Build history of the part. All positions in model axes, mm. A direction names the side the tool comes from. Round coordinates to 2 decimals unless told otherwise and drop trailing zeros. Loops run counter-clockwise (first coordinate to the right, second up) from the corner with the lowest first, then second, coordinate; pieces in that order, holes last. Notation, with made-up numbers: (89.5, 19.25) - (129.5, 19.25) arc R37 ccw to (129.5, 55.25) - close; hole circle Ø4 at (-18, 17.25). An arc over 180 degrees is marked (long way). Use a Markdown table: item, result.
from build123d import *
from build123d.topology import SkipClean

# Parameters (mm, degrees)
BOSS_EXTRUDE1_DEPTH = 2
SKETCH4_R           = 1
CUT_EXTRUDE3_DEPTH  = 2
SKETCH5_R           = 2
CUT_EXTRUDE4_DEPTH  = 1
SKETCH2_R           = 5
CUT_EXTRUDE1_DEPTH  = 10
SKETCH3_R           = 24
CUT_EXTRUDE2_DEPTH  = 10
BOSS_EXTRUDE2_START = 7.2
SKETCH6_R           = 28
SKETCH6_R_2         = 24
BOSS_EXTRUDE2_DEPTH = 7.2
SKETCH7_R           = 28
SKETCH7_R_2         = 14
BOSS_EXTRUDE3_DEPTH = 2
SKETCH9_W           = 14
SKETCH9_H           = 12
BOSS_EXTRUDE4_DEPTH = 4
FILLET1_R           = 7
SKETCH10_R          = 3.25
CUT_EXTRUDE6_DEPTH  = 3
BOSS_EXTRUDE5_DEPTH = 2
FILLET2_R           = 7
FILLET3_R           = 7
FILLET4_R           = 4
FILLET5_R           = 4
SKETCH12_W          = 15
SKETCH12_H          = 7
CUT_EXTRUDE7_DEPTH  = 10


# Some blends are built 0.0001 mm under size
with BuildPart() as part:
    # Sketch1 → Boss-Extrude1 (new body)
    with BuildSketch(Plane(origin=(0, 0, 0), x_dir=(1, 0, 0), z_dir=(0, 1, 0))):
        with BuildLine():
            Line((-37.46998799, 30), (37.46998799, 30))
            ThreePointArc((37.46998799, 30), (0, -48), (-37.46998799, 30))
        make_face()
    extrude(amount=BOSS_EXTRUDE1_DEPTH)

    # Sketch4 → Cut-Extrude3 (cut)
    with BuildSketch(Plane(origin=(0, 2, 0), x_dir=(1, 0, 0), z_dir=(0, 1, 0))):
        with Locations(Location((-44.167045026, 13, 0), (0, 0, 270))):
            Circle(SKETCH4_R)
        with Locations(Location((0, -46.347801012, 0), (0, 0, 270))):
            Circle(SKETCH4_R)
        with Locations(Location((44.167045026, 13, 0), (0, 0, 270))):
            Circle(SKETCH4_R)
    extrude(amount=-CUT_EXTRUDE3_DEPTH, mode=Mode.SUBTRACT)

    # Sketch5 → Cut-Extrude4 (cut)
    with BuildSketch(Plane(origin=(0, 2, 0), x_dir=(1, 0, 0), z_dir=(0, 1, 0))):
        with Locations((-44.167045026, 13)):
            Circle(SKETCH5_R)
        with Locations((0, -46.347801012)):
            Circle(SKETCH5_R)
        with Locations((44.167045026, 13)):
            Circle(SKETCH5_R)
    extrude(amount=-CUT_EXTRUDE4_DEPTH, mode=Mode.SUBTRACT)

    # Sketch2 → Cut-Extrude1 (cut)
    with BuildSketch(Plane(origin=(0, 2, 0), x_dir=(1, 0, 0), z_dir=(0, 1, 0))):
        with Locations(Location((1.35, 0.05, 0), (0, 0, 270))):
            Circle(SKETCH2_R)
    extrude(amount=-CUT_EXTRUDE1_DEPTH, mode=Mode.SUBTRACT)

    # Sketch3 → Cut-Extrude2 (cut)
    with BuildSketch(Plane(origin=(0, 2, 0), x_dir=(1, 0, 0), z_dir=(0, 1, 0))):
        with Locations(Location((1.35, 0.05, 0), (0, 0, 270))):
            Circle(SKETCH3_R)
    extrude(amount=-CUT_EXTRUDE2_DEPTH, mode=Mode.SUBTRACT)

    # Sketch6 → Boss-Extrude2 (add)
    with BuildSketch(Plane(origin=(0, 2, 0), x_dir=(1, 0, 0), z_dir=(0, 1, 0)).offset(BOSS_EXTRUDE2_START)):
        with Locations(Location((1.35, 0.05, 0), (0, 0, 270))):
            Circle(SKETCH6_R)
        with Locations(Location((1.35, 0.05, 0), (0, 0, 270))):
            Circle(SKETCH6_R_2, mode=Mode.SUBTRACT)
    extrude(amount=-BOSS_EXTRUDE2_DEPTH)

    # Sketch7 → Boss-Extrude3 (add)
    with BuildSketch(Plane(origin=(0, 9.2, 0), x_dir=(1, 0, 0), z_dir=(0, 1, 0))):
        with Locations(Location((1.35, 0.05, 0), (0, 0, 270))):
            Circle(SKETCH7_R)
        with Locations(Location((1.35, 0.05, 0), (0, 0, 270))):
            Circle(SKETCH7_R_2, mode=Mode.SUBTRACT)
    extrude(amount=-BOSS_EXTRUDE3_DEPTH)

    # Sketch9 → Boss-Extrude4 (add)
    with BuildSketch(Plane(origin=(0, 0, -30), x_dir=(-1, 0, 0), z_dir=(0, 0, -1))):
        with Locations((-22.46998799, -4)):
            Rectangle(SKETCH9_W, SKETCH9_H)
        with Locations((22.46998799, -4)):
            Rectangle(SKETCH9_W, SKETCH9_H)
    extrude(amount=-BOSS_EXTRUDE4_DEPTH)

    # Fillet1
    fillet1_edges = [part.edges().sort_by_distance(p)[0] for p in [
        (-29.46998799, -10, -28),
        (-15.46998799, -10, -28),
        (15.46998799, -10, -28),
        (29.46998799, -10, -28),
    ]]
    fillet(fillet1_edges, radius=FILLET1_R - 0.0001)  # a hair under: the kernel refuses the full size

    # Sketch10 → Cut-Extrude6 (cut)
    with BuildSketch(Plane(origin=(0, 0, -30), x_dir=(-1, 0, 0), z_dir=(0, 0, -1))):
        with Locations((-22.46998799, -3)):
            Circle(SKETCH10_R)
        with Locations((22.46998799, -3)):
            Circle(SKETCH10_R)
    extrude(amount=-CUT_EXTRUDE6_DEPTH, mode=Mode.SUBTRACT)

    # Sketch11 → Boss-Extrude5 (add)
    with BuildSketch(Plane(origin=(0, 9.2, 0), x_dir=(1, 0, 0), z_dir=(0, 1, 0))):
        with BuildLine():
            Line((-8.65, 15.016629547), (-8.65, 9.847958971))
            ThreePointArc((-8.65, 9.847958971), (1.35, 14.05), (11.35, 9.847958971))
            Line((11.35, 9.847958971), (11.35, 15.016629547))
            ThreePointArc((11.35, 15.016629547), (1.35, 18.05), (-8.65, 15.016629547))
        make_face()
    extrude(amount=-BOSS_EXTRUDE5_DEPTH)

    # Fillet2
    fillet2_edges = [part.edges().sort_by_distance(p)[0] for p in [
        (1.35, 9.2, -28.05),
    ]]
    fillet(fillet2_edges, radius=FILLET2_R)

    # Fillet3
    # the kernel refuses this fillet: 7 mm, written as the material it takes off along each edge
    with BuildSketch(Plane(origin=(1.35, 9.2, -0.05), x_dir=(0, 0, 1), z_dir=(-1, 0, 0))) as fillet3_piece_1:
        with BuildLine():
            CenterArc((18.898979486, -7), FILLET3_R, 90, 44.415308597)
            Line((14, -2), (13.90202041, -1.9))
            ThreePointArc((13.90202041, -1.9), (13.86, -1), (13.86, 0))
            Line((13.86, 0), (14, 0.14))
            Line((14, 0.14), (18.898979486, 0.14))
            Line((18.898979486, 0.14), (18.898979486, 0))
        make_face()
    revolve(axis=Axis((1.35, 9.2, -0.05), (0, 1, 0)), revolution_arc=134.415308597, mode=Mode.SUBTRACT)
    with BuildSketch(Plane(origin=(1.35, 9.2, -0.05), x_dir=(-0.7142857142857139, 0, -0.6998542122237655), z_dir=(0.6998542122237655, 0, -0.7142857142857139))) as fillet3_piece_2:
        with BuildLine():
            CenterArc((18.898979486, -7), FILLET3_R, 90, 44.415308597)
            Line((14, -2), (13.90202041, -1.9))
            ThreePointArc((13.90202041, -1.9), (13.86, -1), (13.86, 0))
            Line((13.86, 0), (14, 0.14))
            Line((14, 0.14), (18.898979486, 0.14))
            Line((18.898979486, 0.14), (18.898979486, 0))
        make_face()
    revolve(axis=Axis((1.35, 9.2, -0.05), (0, 1, 0)), revolution_arc=134.415308597, mode=Mode.SUBTRACT)
    with BuildSketch(Plane(origin=(1.35, 9.2, -0.05), x_dir=(-0.7142857142857144, 0, -0.6998542122237652), z_dir=(-0.6998542122237652, 0, 0.7142857142857144))) as fillet3_piece_3:
        with BuildLine():
            CenterArc((18.898979486, 7), FILLET3_R, 225.584691403, 44.415308597)
            Line((14, 2), (13.90202041, 1.9))
            ThreePointArc((13.90202041, 1.9), (13.86, 1), (13.86, 0))
            Line((13.86, 0), (14, -0.14))
            Line((14, -0.14), (18.898979486, -0.14))
            Line((18.898979486, -0.14), (18.898979486, 0))
        make_face()
    revolve(axis=Axis((1.35, 9.2, -0.05), (0, -1, 0)), revolution_arc=91.169382806, mode=Mode.SUBTRACT)

    # Fillet4
    fillet4_edges = [part.edges().sort_by_distance(p)[0] for p in [
        (1.35, 7.2, -24.05),
    ]]
    fillet(fillet4_edges, radius=FILLET4_R)

    # Fillet5
    fillet5_edges = [part.edges().sort_by_distance(p)[0] for p in [
        (1.35, 0, -24.05),
    ]]
    fillet(fillet5_edges, radius=FILLET5_R)

    # Sketch12 → Cut-Extrude7 (cut)
    with SkipClean():  # the faces are left unmerged after this step: merging them gives an invalid solid
        with BuildSketch(Plane(origin=(0, 2, 0), x_dir=(1, 0, 0), z_dir=(0, 1, 0))):
            with Locations((0, -33.666351983)):
                Rectangle(SKETCH12_W, SKETCH12_H)
        extrude(amount=-CUT_EXTRUDE7_DEPTH, mode=Mode.SUBTRACT)


solid = part.part
Q1. Cut at B-B, the plane x = 35. List the corners of the cut face in (y, z), plus the area to 3 significant figures.
Results found:
| item | result |
|---|---|
| outline | (0, -30) - (2, -30) - (2, 32.85) - (0, 32.85) - close |
| area | 126 mm2 |
Q2. Cut at C-C, the plane y = 6. List the corners of the cut face in (x, z), plus the area to 3 significant figures.
Results found:
| item | result |
|---|---|
| outline | circle Ø53.76 at (1.35, -0.05); hole circle Ø45.71 at (1.35, -0.05) |
| area | 628 mm2 |
Q3. Probe line 1 (Z direction, x = 0, y = 1.7); line 2 (Y direction, x = -26.5, z = -20); line 3 (Z direction, x = 0, y = 1.4). List the from-to ranges inside material, lowest first.
Results found:
| item | result |
|---|---|
| line 1 | z = -30 to -24.7, 24.6 to 30.17, 37.17 to 44.35 |
| line 2 | y = 0 to 2 |
| line 3 | z = -30 to -24.93, 24.83 to 30.17, 37.17 to 44.35 |
Q4. Drop flat-ended pins along their axis: pin 1 (5 mm diameter, centred on x = -0.5, y = 3, fed in from +Z); pin 2 (2 mm diameter, centred on x = 43.5, z = -13.5, fed in from +Y); pin 3 (1.6 mm diameter, centred on x = 0, z = 46.35, fed in from +Y); pin 4 (3 mm diameter, centred on x = -13.5, y = 1, fed in from +Z). Give the stop position or say it passes through.
Results found:
| item | result |
|---|---|
| pin 1 | stops at z = 48 |
| pin 2 | stops at y = 1 |
| pin 3 | passes through |
| pin 4 | stops at z = 46.48 |
Q5. Which spindle directions (+Z, -Z, +X, -X, +Y, -Y) get a long thin tool onto all of the face, cutting with end or side? Do faces 4 (the face through (0, 1, 45)), 5 (the face through (-7.5, 1, 34)), 6 (the face through (23, -3, -27)), 7 (the face through (17.57, -8, -27.97)), 8 (the face through (-29.47, -2, -28)). Say none if no direction does.
Results found:
| item | result |
|---|---|
| face 4 | +Y |
| face 5 | +Y, -Y |
| face 6 | -Z |
| face 7 | +Z, -Z, -Y |
| face 8 | +Z, -Z, -X, -Y |
Q6. Pull direction Z, two halves, no side cores. Call faces 1 (the face through (-45.143, 0.507, -13.217)), 2 (the face through (5, 9.2, -19)), 3 (the face through (-22, -3, -27)): pulls with the +Z half, pulls with the -Z half, needs draft (parallel to the pull), parting line crosses it, or undercut.
Results found:
| item | result |
|---|---|
| face 1 | undercut |
| face 2 | needs draft |
| face 3 | pulls with the -Z half |
Q7. Cut at A-A, the plane y = -4.75. List the corners of the cut face in (x, z).
Results found:
| item | result |
|---|---|
| outline | (-29.25, -30) - (-25.21, -30) - (-25.21, -27) - (-19.73, -27) - (-19.73, -30) - (-15.69, -30) - (-15.69, -26) - (-29.25, -26) - close; (15.69, -30) - (19.73, -30) - (19.73, -27) - (25.21, -27) - (25.21, -30) - (29.25, -30) - (29.25, -26) - (15.69, -26) - close |
